For this review, take the finished solid that the model builds, in its own axes (mm). A direction names the side the tool comes from. Give positions to 0.01 mm unless a question says otherwise; leave off trailing zeros. Order: outer loops, then holes, each group sorted by start corner. A loop starts at its lowest first (then second) coordinate and runs counter-clockwise, first axis right, second up. Notation, with made-up numbers: (-10, 40) - (31, 40) arc R22 cw to (31, 58) - close; hole circle Ø5 at (49, 2.5). An arc over 180 degrees is marked (long way). One line per item, written item: value.
```python
from build123d import *

# Parameters (mm, degrees)
SKETCH_1_R          = 2.75
EXTRUDE_1_DEPTH     = 3
SKETCH_2_R          = 1.5
EXTRUDE_2_DEPTH     = 6
CUT_EXTRUDE_1_DEPTH = 1.3


with BuildPart() as part:
    # 草图1 → 凸台-拉伸1 (new body)
    with BuildSketch(Plane(origin=(0, 0, 0), x_dir=(1, 0, 0), z_dir=(0, 1, 0))):
        Circle(SKETCH_1_R)
    extrude(amount=EXTRUDE_1_DEPTH)

    # 草图2 → 凸台-拉伸2 (add)
    with BuildSketch(Plane(origin=(0, 3, 0), x_dir=(1, 0, 0), z_dir=(0, 1, 0))):
        Circle(SKETCH_2_R)
    extrude(amount=EXTRUDE_2_DEPTH)

    # 草图3 → 切除-拉伸1 (cut)
    with BuildSketch(Plane.XZ):
        Polygon((0.743601936, 1.290680503), (-0.745961136, 1.289318418), (-1.489563072, -0.001362085), (-0.743601936, -1.290680503), (0.745961136, -1.289318418), (1.489563072, 0.001362085), align=None)
    extrude(amount=-CUT_EXTRUDE_1_DEPTH, mode=Mode.SUBTRACT)


solid = part.part
```
(1) Take a section at C-C (y = 5). Write out the cut boundary in (x, z).
Answers below:
outline: circle Ø3 at (0, 0)
(2) Take a section at D-D (x = -2). Write out the cut boundary in (y, z), then the cut area to 3 significant figures.
Answers below:
outline: (0, -1.89) - (3, -1.89) - (3, 1.89) - (0, 1.89) - close
area: 11.3 mm^2
(3) Draft analysis for pull direction X (two halves, no side actions). For faces 4 (the face through (-1.113, 0.641, 0.653)), 5 (the face through (-1.5, 5.96, -0.07)), 6 (the face through (1.2, 0, 1.2)), state which applies: pulls with the +X half, pulls with the -X half, needs draft (parallel to the pull), parting line crosses it, or undercut.
Answers below:
face 4: undercut
face 5: parting line crosses it
face 6: needs draft
(4) Take a section at B-B (z = 0.2). Write out the cut boundary in (x, y), then the cut area to 3 significant figures.
Answers below:
outline: (-2.74, 0) - (-1.37, 0) - (-1.37, 1.3) - (1.37, 1.3) - (1.37, 0) - (2.74, 0) - (2.74, 3) - (1.49, 3) - (1.49, 9) - (-1.49, 9) - (-1.49, 3) - (-2.74, 3) - close
area: 30.7 mm^2
(5) Machinability: for faces 1 (the face through (1.2, 3, 1.2)), 2 (the face through (-0.596, 1.479, 2.685)), 3 (the face through (1.12, 0.64, 0.64)), which of the approach directions +Z, -Z, +X, -X, +Y, -Y give a long, thin tool a straight path to every point of the face, cutting with its end or side? Answer none if there is none.
Answers below:
face 1: +Y
face 2: +Y, -Y
face 3: -Y
(6) Take a section at A-A (x = -0.55). Write out the cut boundary in (y, z), then the cut area to 3 significant figures.
Answers below:
outline: (0, -2.69) - (3, -2.69) - (3, -1.4) - (9, -1.4) - (9, 1.4) - (3, 1.4) - (3, 2.69) - (0, 2.69) - (0, 1.29) - (1.3, 1.29) - (1.3, -1.29) - (0, -1.29) - close
area: 29.6 mm^2
(7) Wall thickness on line 1 (Y direction, x = 2, z = -0.55); line 2 (X direction, y = 6.75, z = -0.05); line 3 (Z direction, x = 0.4, y = 0.5): over which ranges is each line inside the solid? List them lowest first. Write a range as from..to.
Answers below:
line 1: y = 0..3
line 2: x = -1.5..1.5
line 3: z = -2.72..-1.29, 1.29..2.72
